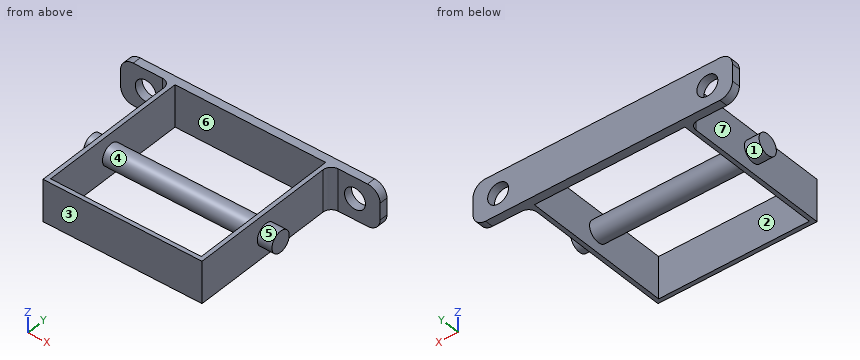
```python
from build123d import *

# Parameters (mm, degrees)
SKETCH1_W           = 96.52
SKETCH1_H           = 96.52
SKETCH1_W_2         = 91.44
SKETCH1_H_2         = 91.44
BOSS_EXTRUDE1_DEPTH = 25.4
SKETCH3_W           = 157.48
SKETCH3_H           = 25.4
BOSS_EXTRUDE2_DEPTH = 2.54
FILLET1_R           = 5.08
SKETCH4_R           = 6.35
CUT_EXTRUDE2_DEPTH  = 161.02
FILLET2_R           = 7.62
SKETCH5_R           = 6.35
BOSS_EXTRUDE4_DEPTH = 57.15


with BuildPart() as part:
    # Sketch1 → Boss-Extrude1 (new body)
    with BuildSketch(Plane.XY):
        with Locations((48.26, -48.26)):
            Rectangle(SKETCH1_W, SKETCH1_H)
        with Locations((48.26, -48.26)):
            Rectangle(SKETCH1_W_2, SKETCH1_H_2, mode=Mode.SUBTRACT)
    extrude(amount=BOSS_EXTRUDE1_DEPTH)

    # Sketch3 → Boss-Extrude2 (add, symmetric)
    with BuildSketch(Plane(origin=(0, 0, 0), x_dir=(1, 0, 0), z_dir=(0, 1, 0))):
        with Locations((48.26, -12.7)):
            Rectangle(SKETCH3_W, SKETCH3_H)
    extrude(amount=BOSS_EXTRUDE2_DEPTH, both=True)

    # Fillet1
    fillet1_edges = [part.edges().sort_by_distance(p)[0] for p in [
        (0, -2.54, 12.7),
        (96.52, -2.54, 12.7),
    ]]
    fillet(fillet1_edges, radius=FILLET1_R)

    # Sketch4 → Cut-Extrude2 (cut, through all)
    with BuildSketch(Plane.XZ.offset(2.54)):
        with Locations(Location((111.76, 12.7, 0), (0, 0, 270))):
            Circle(SKETCH4_R)
        with Locations(Location((-15.24, 12.7, 0), (0, 0, 90))):
            Circle(SKETCH4_R)
    extrude(amount=-CUT_EXTRUDE2_DEPTH, mode=Mode.SUBTRACT)

    # Fillet2
    fillet2_edges = [part.edges().sort_by_distance(p)[0] for p in [
        (-30.48, 0, 25.4),
        (127, 0, 0),
        (-30.48, 0, 0),
        (127, 0, 25.4),
    ]]
    fillet(fillet2_edges, radius=FILLET2_R)

    # Sketch5 → Boss-Extrude4 (add, symmetric)
    with BuildSketch(Plane(origin=(48.26, 0, 0), x_dir=(0, 0, -1), z_dir=(1, 0, 0))):
        with Locations(Location((-12.7, -49.53, 0), (0, 0, 270))):
            Circle(SKETCH5_R)
    extrude(amount=BOSS_EXTRUDE4_DEPTH, both=True)


solid = part.part
```
Here's how the part is built. I have some questions about the finished solid (model axes, mm). Face numbers are marked on the shaded views. A direction names the side the tool comes from. Coordinates: 2 decimals unless noted, no trailing zeros. Order: outer loops, then holes, each group sorted by start corner. A loop starts at its lowest first (then second) coordinate and runs counter-clockwise, first axis right, second up.
Item 1: If we section it at A-A, the plane z = 12.7: Give the number of separate pieces and of enclosed holes in the cut face, then the cut area to 3 significant figures.
Response values:
separate pieces: 3
enclosed holes: 2
area: 2,780 mm2
Item 2: I'm going to push flat-ended pins straight in: pin 1 Ø7.5 at (y, z) = (-62, 14) entering from -X; pin 2 Ø1 at (x, y) = (76, -41) entering from -Z; pin 3 Ø14.5 at (x, z) = (111.76, 12.7) entering from -Y; pin 4 Ø10 at (y, z) = (-48.5, 11.5) entering from +X. Where does each tip first touch, or does it pass through?
Response values:
pin 1: stops at x = 0
pin 2: passes through
pin 3: stops at y = -55.88
pin 4: stops at x = 105.41
Item 3: Which directions (+Z, -Z, +X, -X, +Y, -Y) give clear straight access to the entire face, cutting with the end or side of a thin tool? Please do the marked faces 1, 2, 3 and 4.
Response values:
face 1: -X
face 2: +Z, -Z
face 3: +Z, -Z, +X, -X, -Y
face 4: none
Item 4: If we section it at D-D, the plane x = -15.24: List the corners of the cut face in (y, z) for me, then the cut area to 3 significant figures.
Response values:
outline: (-2.54, 0) - (2.54, 0) - (2.54, 6.35) - (-2.54, 6.35) - close; (-2.54, 19.05) - (2.54, 19.05) - (2.54, 25.4) - (-2.54, 25.4) - close
area: 64.5 mm2
Item 5: If we section it at B-B, the plane x = 17.5: List the corners of the cut face in (y, z) for me.
Response values:
outline: (-96.52, 0) - (-93.98, 0) - (-93.98, 25.4) - (-96.52, 25.4) - close; circle Ø12.7 at (-49.53, 12.7); (-2.54, 0) - (2.54, 0) - (2.54, 25.4) - (-2.54, 25.4) - close
Item 6: Thinking about a two-plate mould opening in X: for the marked faces 5, 6 and 7, which applies, pulls with the +X half, pulls with the -X half, needs draft (parallel to the pull), parting line crosses it, or undercut?
Response values:
face 5: needs draft
face 6: undercut
face 7: pulls with the -X half
Item 7: I need wall thicknesses on probe 1 along X at (y, z) = (-0.6, 12.7); probe 2 along X at (y, z) = (-39, 8.25); probe 3 along Y at (x, z) = (80.5, 9.5). Which ranges of each line are inside material? Lowest first, please.
Response values:
probe 1: x = -30.48 to -21.59, -8.89 to 105.41, 118.11 to 127
probe 2: x = 0 to 2.54, 93.98 to 96.52
probe 3: y = -96.52 to -93.98, -55.01 to -44.05, -2.54 to 2.54
Item 8: If we section it at C-C, the plane y = -83: List the corners of the cut face in (x, z) for me, then the cut area to 3 significant figures.
Response values:
outline: (0, 0) - (2.54, 0) - (2.54, 25.4) - (0, 25.4) - close; (93.98, 0) - (96.52, 0) - (96.52, 25.4) - (93.98, 25.4) - close
area: 129 mm2
